```python
from build123d import *

# Parameters (mm, degrees)
F1_DEPTH = 25
F2_DEPTH = 2


with BuildPart() as f1:
    # F0 (on Top) → F1 (new body)
    with BuildSketch(Plane.XY):
        with BuildLine():
            ThreePointArc((-19.5, 24.5), (-23.035534, 23.035534), (-24.5, 19.5))
            Line((-24.5, 19.5), (-24.5, -19.5))
            ThreePointArc((-24.5, -19.5), (-23.035534, -23.035534), (-19.5, -24.5))
            Line((-19.5, -24.5), (19.5, -24.5))
            ThreePointArc((19.5, -24.5), (23.035534, -23.035534), (24.5, -19.5))
            Line((24.5, -19.5), (24.5, 19.5))
            ThreePointArc((24.5, 19.5), (23.035534, 23.035534), (19.5, 24.5))
            Line((19.5, 24.5), (-19.5, 24.5))
        make_face()
        with BuildLine():
            Line((-22.1, -19.5), (-22.1, 19.5))
            ThreePointArc((-22.1, 19.5), (-21.338478, 21.338478), (-19.5, 22.1))
            Line((-19.5, 22.1), (19.5, 22.1))
            ThreePointArc((19.5, 22.1), (21.338478, 21.338478), (22.1, 19.5))
            Line((22.1, 19.5), (22.1, -19.5))
            ThreePointArc((22.1, -19.5), (21.338478, -21.338478), (19.5, -22.1))
            Line((19.5, -22.1), (-19.5, -22.1))
            ThreePointArc((-19.5, -22.1), (-21.338478, -21.338478), (-22.1, -19.5))
        make_face(mode=Mode.SUBTRACT)
    extrude(amount=F1_DEPTH)

    # F0 (on Top) → F2 (join)
    with BuildSketch(Plane.XY):
        with BuildLine():
            ThreePointArc((-19.5, 22.1), (-21.338478, 21.338478), (-22.1, 19.5))
            Line((-22.1, 19.5), (-22.1, -19.5))
            ThreePointArc((-22.1, -19.5), (-21.338478, -21.338478), (-19.5, -22.1))
            Line((-19.5, -22.1), (19.5, -22.1))
            ThreePointArc((19.5, -22.1), (21.338478, -21.338478), (22.1, -19.5))
            Line((22.1, -19.5), (22.1, 19.5))
            ThreePointArc((22.1, 19.5), (21.338478, 21.338478), (19.5, 22.1))
            Line((19.5, 22.1), (-19.5, 22.1))
        make_face()
    extrude(amount=F2_DEPTH)


solid = f1.part
```
Geometry check sheet. Reference: the model listing, model coordinates, mm. A direction names the side the tool comes from. Round coordinates to 2 decimals unless told otherwise and drop trailing zeros. Order: outer loops, then holes, each group sorted by start corner. A loop starts at its lowest first (then second) coordinate and runs counter-clockwise, first axis right, second up. Notation, with made-up numbers: (18.25, 19) - (55.25, 19) arc R14 cw to (55.25, 31) - close; hole circle Ø2 at (58.5, -14). An arc over 180 degrees is marked (long way). Use a Markdown table: item, result. Add a question column.
1) Gauge pin test, flat ends, axial feed: P1, Ø13.5, axis at x = -4.5, y = 9, coming from the +Z side; P2, Ø12, axis at x = -5, y = 3, coming from the -Z side. Record the tip position at first contact, or that the pin passes through.
2) Set-up check for faces 4 (the flat face through (-22.1, 0, 13)), 5 (the flat face through (0, 0, 0)): record each of +Z, -Z, +X, -X, +Y, -Y from which the full face is reachable in a straight line by a thin tool's end or side.
3) Mould release check, pull along Y, two halves, no side actions. Record for faces 1 (the cylindrical face through (-21.318, -21.359, 13.339)), 2 (the flat face through (0, -24.5, 12)), 3 (the flat face through (-24.5, 0, 12)): released by +Y, released by -Y, zero draft, split by the parting line, or undercut.
4) Thickness scan on line 1 along X through (y, z) = (-1.5, 9.75); line 2 along Z through (x, y) = (5, -17). Record the ranges inside material, lowest first.
5) Section check B-B (y = -13.5). Record the cut outline in (x, z).
6) Section check A-A (z = 16.25). Record the cut outline in (x, y), then the cut area to 3 significant figures.
Established:
| question | item | result |
|---|---|---|
| 1 | P1 | z = 2 |
| 1 | P2 | z = 0 |
| 2 | face 4 | +Z |
| 2 | face 5 | -Z, +X, -X, +Y, -Y |
| 3 | face 1 | undercut |
| 3 | face 2 | released by -Y |
| 3 | face 3 | zero draft |
| 4 | line 1 | -24.5 to -22.1, 22.1 to 24.5 |
| 4 | line 2 | 0 to 2 |
| 5 | outline | (-24.5, 0) - (24.5, 0) - (24.5, 25) - (22.1, 25) - (22.1, 2) - (-22.1, 2) - (-22.1, 25) - (-24.5, 25) - close |
| 6 | outline | (-24.5, -19.5) arc R5 ccw to (-19.5, -24.5) - (19.5, -24.5) arc R5 ccw to (24.5, -19.5) - (24.5, 19.5) arc R5 ccw to (19.5, 24.5) - (-19.5, 24.5) arc R5 ccw to (-24.5, 19.5) - close; hole (-22.1, -19.5) arc R2.6 ccw to (-19.5, -22.1) - (19.5, -22.1) arc R2.6 ccw to (22.1, -19.5) - (22.1, 19.5) arc R2.6 ccw to (19.5, 22.1) - (-19.5, 22.1) arc R2.6 ccw to (-22.1, 19.5) - close |
| 6 | area | 432 mm2 |
